For this review, take the finished solid that the model builds, in its own axes (mm). Face numbers are marked on the shaded views. A direction names the side the tool comes from. Coordinates: 2 decimals unless noted, no trailing zeros. Write each loop counter-clockwise with the first axis right and the second up, starting at its lowest first coordinate (ties: lowest second). Pieces come first, ordered by that corner, then holes. Notation, with made-up numbers: (5, 71) -> (63, 71) arc R21 cw to (63, 105) -> close; hole circle Ø5 at (40, 86.5). An arc over 180 degrees is marked (long way). Put each result on its own line as item: value. Start each with the question number.
Item 1: For the marked faces 1, 2 and 3, list the 3-axis set-ups (+Z, -Z, +X, -X, +Y, -Y) from which the entire face can be reached by the end or side of a thin tool; tool diameter is ignored.
Item 2: Consider section B-B on x = 63.5. Give the boundary of the cut face in (y, z).
Item 3: Consider section A-A on y = 402.5. Give the boundary of the cut face in (x, z), and give its area (3 significant figures).
Item 4: Insertion check: P1, Ø5, axis at y = 303, z = -48.5, coming from the +X side; P2, Ø9.5, axis at y = 623.5, z = 24, coming from the +X side; P3, Ø5, axis at y = 422, z = -42.5, coming from the -X side. Each pin has a flat end and moves straight along its axis. Give the tip position at first contact, or say it passes through.
Item 5: To check wall thickness, follow L1, parallel to Z at x = 181, y = 628.65; L2, parallel to X at y = 595, z = -42.5; L3, parallel to Y at x = 111, z = 16.5. State the ranges of each line that lie inside material, in increasing order.
```python
from build123d import *

# Parameters (mm, degrees)
F0_W     = 419.1
F0_H     = 132.5626
F1_DEPTH = 609.6
F0_W_2   = 31.75
F2_DEPTH = 3.175
F3_W     = 6.35
F3_H     = 38.354
F4_DEPTH = 31.75
F5_R     = 4.7625
F6_DEPTH = 425.451


with BuildPart() as f1:
    # F0 (on Front) → F1 (new body)
    with BuildSketch(Plane.XZ):
        Rectangle(F0_W, F0_H)
    extrude(amount=-F1_DEPTH)

    # F0 (on Front) → F2 (join)
    with BuildSketch(Plane.XZ):
        with Locations((225.425, 0)):
            Rectangle(F0_W_2, F0_H)
        Rectangle(F0_W, F0_H)
        with Locations((-225.425, 0)):
            Rectangle(F0_W_2, F0_H)
    extrude(amount=-F2_DEPTH)

    # F3 (on face) → F4 (join)
    with BuildSketch(Plane(origin=(0, 609.6, 0), x_dir=(-1, 0, 0), z_dir=(0, 1, 0))):
        with Locations((-180.975, 31.7373)):
            Rectangle(F3_W, F3_H)
        with Locations((-180.975, -19.0627)):
            Rectangle(F3_W, F3_H)
    extrude(amount=F4_DEPTH)

    # F5 (on face) → F6 (cut, through all)
    with BuildSketch(Plane.YZ.offset(184.15)):
        with Locations((628.65, 31.7373)):
            Circle(F5_R)
        with Locations((628.65, -19.0627)):
            Circle(F5_R)
    extrude(amount=-F6_DEPTH, mode=Mode.SUBTRACT)


solid = f1.part
```
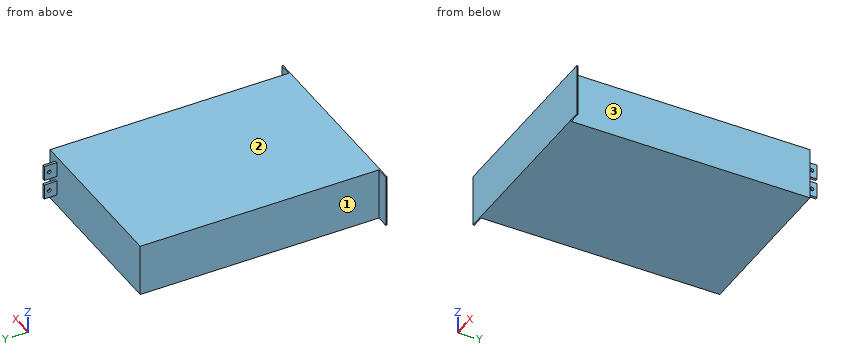
Return value:
1. face 1: +Z, -Z, -X, +Y
1. face 2: +Z, +X, -X, +Y, -Y
1. face 3: +Z, -Z, +X, +Y
2. outline: (0, -66.28) -> (609.6, -66.28) -> (609.6, 66.28) -> (0, 66.28) -> close
3. outline: (-209.55, -66.28) -> (209.55, -66.28) -> (209.55, 66.28) -> (-209.55, 66.28) -> close
3. area: 55,600 mm^2
4. P1: x = 209.55
4. P2: x = 184.15
4. P3: x = -209.55
5. L1: -38.24 to -23.83, -14.3 to 0.11, 12.56 to 26.97, 36.5 to 50.91
5. L2: -209.55 to 209.55
5. L3: 0 to 609.6
